from build123d import *

# Parameters (mm, degrees)
SKETCH_2_W                  = 70
SKETCH_2_H                  = 30
SM_BASE_FLANGE_1_DEPTH      = 1.5
OTHER_START                 = -15
OTHER_1_DEPTH               = 30
OTHER_1_2_DEPTH             = 30
HOLE_WIZARD_M4_1_AT_2_COUNT = 2
HOLE_WIZARD_M4_1_AT_2_PITCH = 55


# Read off the part's stored shape, not the designer's step: 褶边1
# Sheet-metal steps are written as plain solids
with BuildPart() as part:
    # 草图2 → 基体-法兰1 (new body)
    with BuildSketch(Plane.XY):
        Rectangle(SKETCH_2_W, SKETCH_2_H)
    extrude(amount=-SM_BASE_FLANGE_1_DEPTH)

    # Other 1 outline → Other 1 (cut)
    with BuildSketch(Plane(origin=(0, 0, 0), x_dir=(1, 0, 0), z_dir=(0, 1, 0)).offset(OTHER_START)):
        with BuildLine():
            Line((35, 1.5), (34.999193338, 1.5))
            ThreePointArc((34.999193338, 1.5), (34.528192933, 0.436447127), (33.45, 0))
            Line((33.45, 0), (35, 0))
            Line((35, 0), (35, 1.5))
        make_face()
        with BuildLine():
            ThreePointArc((-33.45, 0), (-34.528192933, 0.436447127), (-34.999193338, 1.5))
            Line((-34.999193338, 1.5), (-35, 1.5))
            Line((-35, 1.5), (-35, 0))
            Line((-35, 0), (-33.45, 0))
        make_face()
    extrude(amount=OTHER_1_DEPTH, mode=Mode.SUBTRACT)

    # Other 1 2 outline → Other 1 2 (add)
    with BuildSketch(Plane(origin=(0, 0, 0), x_dir=(1, 0, 0), z_dir=(0, 1, 0)).offset(OTHER_START)):
        with BuildLine():
            Line((23, 3.1), (23, 1.6))
            Line((23, 1.6), (33.45, 1.6))
            ThreePointArc((33.45, 1.6), (33.5, 1.55), (33.45, 1.5))
            Line((33.45, 1.5), (34.999193338, 1.5))
            ThreePointArc((34.999193338, 1.5), (34.563552873, 2.628192933), (33.45, 3.1))
            Line((33.45, 3.1), (23, 3.1))
        make_face()
        with BuildLine():
            Line((-34.999193338, 1.5), (-33.45, 1.5))
            ThreePointArc((-33.45, 1.5), (-33.5, 1.55), (-33.45, 1.6))
            Line((-33.45, 1.6), (-23, 1.6))
            Line((-23, 1.6), (-23, 3.1))
            Line((-23, 3.1), (-33.45, 3.1))
            ThreePointArc((-33.45, 3.1), (-34.563552873, 2.628192933), (-34.999193338, 1.5))
        make_face()
    extrude(amount=OTHER_1_2_DEPTH)

    # 草图9 → M4 六角凹锥坑头螺钉的锥形沉头孔1 (revolve, cut)
    with BuildSketch(Plane(origin=(27.5, 0, 0), x_dir=(0, -1, 0), z_dir=(1, 0, 0))):
        Polygon((0, 0), (0, 3.1), (2.25, 3.1), (2.25, 2.34), (4.59, 0), align=None)
    hole_wizard_m4_1 = revolve(axis=Axis((27.5, 0, 6.35), (0, 0, -1)), mode=Mode.SUBTRACT)

    # M4 六角凹锥坑头螺钉的锥形沉头孔1 at 2: M4 六角凹锥坑头螺钉的锥形沉头孔1 ×2
    with Locations(*[(-i * HOLE_WIZARD_M4_1_AT_2_PITCH, 0, 0) for i in range(1, HOLE_WIZARD_M4_1_AT_2_COUNT)]):
        add(hole_wizard_m4_1, mode=Mode.SUBTRACT)


solid = part.part
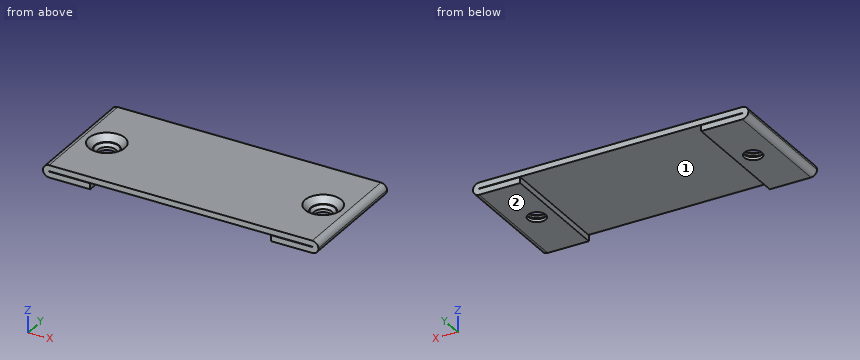
Design review of the part built by this model. Coordinates are the model's own, in mm. Face numbers are marked on the shaded views. Round coordinates to 2 decimals unless told otherwise and drop trailing zeros. Write each loop counter-clockwise with the first axis right and the second up, starting at its lowest first coordinate (ties: lowest second). Pieces come first, ordered by that corner, then holes. Notation, with made-up numbers: (64, 26) - (73, 26) arc R32 cw to (73, 53) - close; hole circle Ø9 at (88.25, 3). An arc over 180 degrees is marked (long way). Use a Markdown table: item, result. Add a question column.
1. Mouldability with a two-part tool opening along X and no side actions: class the marked faces 1 and 2 as +X half, -X half, draft (parallel to the pull), parting line (faces both ways), or undercut.
2. Clearance check with flat-ended pins moving along their axes: pin 1 (2.5 mm diameter, centred on x = -27.5, y = 0, fed in from +Z); pin 2 (1.2 mm diameter, centred on y = -2.5, z = -2.5, fed in from -X); pin 3 (12 mm diameter, centred on x = -9, y = 7.5, fed in from -Z); pin 4 (0.8 mm diameter, centred on y = -7.5, z = -2.5, fed in from +X). State where each tip first meets the part, or that it passes through.
3. We need section A-A (x = 27.5). State the section outline as (y, z) points, then the cut area to 3 significant figures.
4. We need section C-C (y = -7). State the section outline as (x, z) points, then the cut area to 3 significant figures.
5. We need section B-B (y = 0). Count the separate pieces of the cut face and the enclosed holes in it, then the cut area to 3 significant figures.
6. Wall thickness on probe 1 along Y at (x, z) = (27.5, -2.8); probe 2 along X at (y, z) = (1, -2.5); probe 3 along X at (y, z) = (0, -2.8): over which ranges is each line inside the solid? List them lowest first.
Output:
| question | item | result |
|---|---|---|
| 1 | face 1 | undercut |
| 1 | face 2 | draft |
| 2 | pin 1 | passes through |
| 2 | pin 2 | stops at x = -34.96 |
| 2 | pin 3 | stops at z = -1.5 |
| 2 | pin 4 | stops at x = 34.9 |
| 3 | outline | (-15, -3.1) - (-2.25, -3.1) - (-2.25, -2.34) - (-2.99, -1.6) - (-15, -1.6) - close; (-15, -1.5) - (-3.09, -1.5) - (-4.59, 0) - (-15, 0) - close; (2.25, -3.1) - (15, -3.1) - (15, -1.6) - (2.99, -1.6) - (2.25, -2.34) - close; (3.09, -1.5) - (15, -1.5) - (15, 0) - (4.59, 0) - close |
| 3 | area | 71.2 mm2 |
| 4 | outline | (-33.45, -3.1) - (-23, -3.1) - (-23, -1.6) - (-33.45, -1.6) arc R0.05 cw to (-33.45, -1.5) - (33.45, -1.5) arc R0.05 cw to (33.45, -1.6) - (23, -1.6) - (23, -3.1) - (33.45, -3.1) arc R1.55 ccw to (33.45, 0) - (-33.45, 0) arc R1.55 ccw to start |
| 4 | area | 139 mm2 |
| 5 | separate pieces | 5 |
| 5 | enclosed holes | 0 |
| 5 | area | 102 mm2 |
| 6 | probe 1 | y = -15 to -2.25, 2.25 to 15 |
| 6 | probe 2 | x = -34.67 to -29.52, -25.48 to -23, 23 to 25.48, 29.52 to 34.67 |
| 6 | probe 3 | x = -34.37 to -29.75, -25.25 to -23, 23 to 25.25, 29.75 to 34.37 |
